from build123d import *

# Parameters (mm, degrees)
SKETCH_W        = 84.6
SKETCH_H        = 44.6
PAD_DEPTH       = 22.4
SKETCH001_W     = 89.6
SKETCH001_H     = 49.6
PAD001_DEPTH    = 2
FILLET_R        = 0.8
SKETCH002_W     = 51
SKETCH002_H     = 30
POCKET_DEPTH    = 2.82
CHAMFER_SIZE    = 1.5
SKETCH003_R     = 1.81
POCKET001_DEPTH = 3
SKETCH006_W     = 9
SKETCH006_H     = 26
POCKET002_DEPTH = 10
SKETCH007_R     = 1.51
PAD002_DEPTH    = 3


with BuildPart() as part:
    # Sketch → Pad (new body)
    with BuildSketch(Plane.XY):
        Rectangle(SKETCH_W, SKETCH_H)
    extrude(amount=-PAD_DEPTH)

    # Sketch001 → Pad001 (join)
    with BuildSketch(Plane.XY):
        Rectangle(SKETCH001_W, SKETCH001_H)
    extrude(amount=PAD001_DEPTH)

    # Fillet
    fillet_edges = [part.edges().sort_by_distance(p)[0] for p in [
        (0, -24.8, 2),
        (44.8, 0, 2),
        (0, 24.8, 2),
        (-44.8, 0, 2),
    ]]
    fillet(fillet_edges, radius=FILLET_R)

    # Sketch002 (on Face8 of Fillet) → Pocket (cut)
    with BuildSketch(Plane.XY.offset(2)):
        Rectangle(SKETCH002_W, SKETCH002_H)
    extrude(amount=-POCKET_DEPTH, mode=Mode.SUBTRACT)

    # Chamfer
    chamfer_edges = [part.edges().sort_by_distance(p)[0] for p in [
        (-25.5, 0, 2),
        (0, 15, 2),
        (0, -15, 2),
        (25.5, 0, 2),
    ]]
    chamfer(chamfer_edges, length=CHAMFER_SIZE)

    # Sketch003 (on Face1 of Chamfer) → Pocket001 (cut)
    with BuildSketch(Plane.XY.offset(2)):
        with Locations((37, 0)):
            Circle(SKETCH003_R)
    extrude(amount=-POCKET001_DEPTH, mode=Mode.SUBTRACT)

    # Sketch006 (on DatumPlane) → Pocket002 (cut)
    with BuildSketch(Plane.XY.offset(-22.4)):
        with Locations((-37.8, 0)):
            Rectangle(SKETCH006_W, SKETCH006_H)
    extrude(amount=POCKET002_DEPTH, mode=Mode.SUBTRACT)

    # Sketch007 (on DatumPlane) → Pad002 (join)
    with BuildSketch(Plane.XY.offset(-1)):
        with Locations((37, 0)):
            Circle(SKETCH007_R)
    extrude(amount=PAD002_DEPTH)


solid = part.part
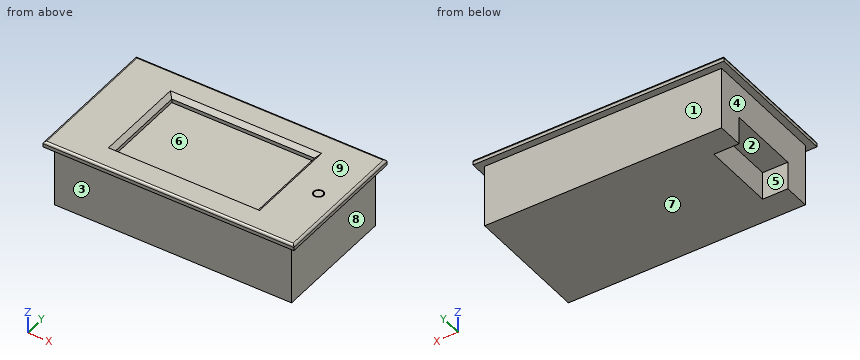
Source: CAD feature listing. Evaluate the final solid. Frame: model axes, mm. Face numbers are marked on the shaded views. A direction names the side the tool comes from. Round coordinates to 2 decimals unless told otherwise and drop trailing zeros. Order: outer loops, then holes, each group sorted by start corner. A loop starts at its lowest first (then second) coordinate and runs counter-clockwise, first axis right, second up. Notation, with made-up numbers: (61, 46.25) - (115, 46.25) arc R30 cw to (115, 70.25) - close; hole circle Ø2 at (49, 46.25). An arc over 180 degrees is marked (long way). Use a Markdown table: item, result. Add a question column.
1. Section query B-B (x = -31). Return the cut outline in (y, z).
2. Section query A-A (y = 0). Return the cut outline in (x, z), then the cut area to 3 significant figures.
3. Line query: probe 1 along Y at (x, z) = (37, 1.35); probe 2 along Z at (x, y) = (-15.5, -12.5); probe 3 along Y at (x, z) = (39, -20). Output: solid intervals per line, ascending.
4. First-contact query: pin 1 (15 mm diameter, centred on x = 3.5, y = -1.5, fed in from +Z); pin 2 (1.1 mm diameter, centred on y = -2.5, z = -0.5, fed in from +X); pin 3 (7 mm diameter, centred on x = -36.5, z = -15.5, fed in from -Y); pin 4 (6 mm diameter, centred on y = 8, z = -6.5, fed in from +X). Flat tips, straight axial feed; report the tip coordinate or a pass-through.
5. Section query C-C (z = -10.25). Return the cut outline in (x, y).
6. Set-up query: the marked faces 5, 6, 7, 8 and 9. Return all of +Z, -Z, +X, -X, +Y, -Y with unobstructed straight access to the full face (end or side cutting, diameter ignored); none if empty.
7. Section query D-D (y = -9). Return the cut outline in (x, z).
8. Mould query, pull axis Y, two halves, no side actions, for the marked faces 1, 2, 3 and 4. Classes: +Y half, -Y half, draft (parallel to the pull), parting line (faces both ways), or undercut.
Derived:
| question | item | result |
|---|---|---|
| 1 | outline | (-24.8, 0) - (-22.3, 0) - (-22.3, -22.4) - (22.3, -22.4) - (22.3, 0) - (24.8, 0) - (24.8, 1.2) arc R0.8 ccw to (24, 2) - (-24, 2) arc R0.8 ccw to (-24.8, 1.2) - close |
| 2 | outline | (-44.8, 0) - (-42.3, 0) - (-42.3, -12.4) - (-33.3, -12.4) - (-33.3, -22.4) - (42.3, -22.4) - (42.3, 0) - (44.8, 0) - (44.8, 1.2) arc R0.8 ccw to (44, 2) - (38.81, 2) - (38.81, -1) - (38.51, -1) - (38.51, 2) - (35.49, 2) - (35.49, -1) - (35.19, -1) - (35.19, 2) - (27, 2) - (25.5, 0.5) - (25.5, -0.82) - (-25.5, -0.82) - (-25.5, 0.5) - (-27, 2) - (-44, 2) arc R0.8 ccw to (-44.8, 1.2) - close |
| 2 | area | 1,840 mm2 |
| 3 | probe 1 | -24.79 to -1.81, -1.51 to 1.51, 1.81 to 24.79 |
| 3 | probe 2 | -22.4 to -0.82 |
| 3 | probe 3 | -22.3 to 22.3 |
| 4 | pin 1 | z = -0.82 |
| 4 | pin 2 | x = 44.8 |
| 4 | pin 3 | y = -22.3 |
| 4 | pin 4 | x = 42.3 |
| 5 | outline | (-42.3, -22.3) - (42.3, -22.3) - (42.3, 22.3) - (-42.3, 22.3) - close |
| 6 | face 5 | -Z, -X |
| 6 | face 6 | +Z |
| 6 | face 7 | -Z, +X, -X, +Y, -Y |
| 6 | face 8 | -Z, +X, +Y, -Y |
| 6 | face 9 | +Z, +X, -X, +Y, -Y |
| 7 | outline | (-44.8, 0) - (-42.3, 0) - (-42.3, -12.4) - (-33.3, -12.4) - (-33.3, -22.4) - (42.3, -22.4) - (42.3, 0) - (44.8, 0) - (44.8, 1.2) arc R0.8 ccw to (44, 2) - (27, 2) - (25.5, 0.5) - (25.5, -0.82) - (-25.5, -0.82) - (-25.5, 0.5) - (-27, 2) - (-44, 2) arc R0.8 ccw to (-44.8, 1.2) - close |
| 8 | face 1 | +Y half |
| 8 | face 2 | undercut |
| 8 | face 3 | -Y half |
| 8 | face 4 | draft |
